Can you work these out from the model? Positions are in its coordinate system, mm. A direction names the side the tool comes from. Give positions to 0.01 mm unless a question says otherwise; leave off trailing zeros. Write each loop counter-clockwise with the first axis right and the second up, starting at its lowest first coordinate (ties: lowest second). Pieces come first, ordered by that corner, then holes.
1. I'm going to push a flat-ended pin straight in: pin 1 (3 mm diameter, centred on x = -42, z = -3.5, fed in from +Y). Where does the tip first touch, or does it pass through?
2. On a 3-axis mill with a long thin cutter (end or side, diameter ignored), from which of +Z, -Z, +X, -X, +Y, -Y can I reach the whole of each face in a straight line? I mean faces 4 (the flat face through (-1, 5, -5)), 5 (the cylindrical face through (-20.966, 10.493, 0.521)). Say none if no direction works.
3. Thinking about a two-plate mould opening in X: for faces 1 (the flat face through (75, 5, 0)), 2 (the cylindrical face through (-64.095, 10.493, 0.867)), 3 (the flat face through (34, 11, 0)), which applies, pulls with the +X half, pulls with the -X half, needs draft (parallel to the pull), parting line crosses it, or undercut?
4. If I drill on probe 1 along Y at (x, z) = (30, 1); probe 2 along Z at (x, y) = (66, 10.25); probe 3 along Z at (x, y) = (67.5, 10.25), over which ranges is the centre line in solid material (lowest first)?
5. Suppose I cut it at B-B (x = -18.5). Please give me the cut outline in (y, z).
6. Suppose I cut it at A-A (x = 51). Please give me the cut outline in (y, z), and give its area (3 significant figures).
```python
from build123d import *

# Parameters (mm, degrees)
SKETCH1_W           = 150
SKETCH1_H           = 10
BOSS_EXTRUDE1_DEPTH = 10
SKETCH2_R           = 4
BOSS_EXTRUDE2_DEPTH = 1


with BuildPart() as part:
    # Sketch1 → Boss-Extrude1 (new body)
    with BuildSketch(Plane(origin=(0, 0, 0), x_dir=(1, 0, 0), z_dir=(0, 1, 0))):
        Rectangle(SKETCH1_W, SKETCH1_H)
    extrude(amount=BOSS_EXTRUDE1_DEPTH)

    # Sketch2 → Boss-Extrude2 (add)
    with BuildSketch(Plane(origin=(0, 10, 0), x_dir=(1, 0, 0), z_dir=(0, 1, 0))):
        with Locations(Location((0, 0, 0), (0, 0, 90))):
            Circle(SKETCH2_R)
        with Locations(Location((17, 0, 0), (0, 0, 90))):
            Circle(SKETCH2_R)
        with Locations(Location((34, 0, 0), (0, 0, 90))):
            Circle(SKETCH2_R)
        with Locations(Location((51, 0, 0), (0, 0, 90))):
            Circle(SKETCH2_R)
        with Locations(Location((68, 0, 0), (0, 0, 90))):
            Circle(SKETCH2_R)
        with Locations(Location((-17, 0, 0), (0, 0, 90))):
            Circle(SKETCH2_R)
        with Locations(Location((-34, 0, 0), (0, 0, 90))):
            Circle(SKETCH2_R)
        with Locations(Location((-51, 0, 0), (0, 0, 90))):
            Circle(SKETCH2_R)
        with Locations(Location((-68, 0, 0), (0, 0, 90))):
            Circle(SKETCH2_R)
    extrude(amount=BOSS_EXTRUDE2_DEPTH)


solid = part.part
```
Checks:
1. pin 1: stops at y = 10
2. face 4: -Z, +X, -X, +Y, -Y
2. face 5: +Y
3. face 1: pulls with the +X half
3. face 2: undercut
3. face 3: needs draft
4. probe 1: y = 0 to 10
4. probe 2: z = -3.46 to 3.46
4. probe 3: z = -3.97 to 3.97
5. outline: (0, -5) - (10, -5) - (10, -3.71) - (11, -3.71) - (11, 3.71) - (10, 3.71) - (10, 5) - (0, 5) - close
6. outline: (0, -5) - (10, -5) - (10, -4) - (11, -4) - (11, 4) - (10, 4) - (10, 5) - (0, 5) - close
6. area: 108 mm2
